from build123d import *

# Parameters (mm, degrees)
SKETCH2_W           = 50
SKETCH2_H           = 50
BOSS_EXTRUDE1_DEPTH = 3.175
SKETCH3_R           = 1.375
CUT_EXTRUDE1_DEPTH  = 36.497614356
SKETCH5_R           = 2.375
CUT_EXTRUDE3_DEPTH  = 1.9
CUT_EXTRUDE9_DEPTH  = 36.497614356
FILLET1_R           = 3
SKETCH11_W          = 15
SKETCH11_H          = 30
BOSS_EXTRUDE2_DEPTH = 3.175
CUT_EXTRUDE10_REACH = 62.499
CHAMFER1_SIZE       = 5


with BuildPart() as part:
    # Sketch2 → Boss-Extrude1 (new body)
    with BuildSketch(Plane(origin=(0, 0, 0), x_dir=(1, 0, 0), z_dir=(0, 1, 0))):
        Rectangle(SKETCH2_W, SKETCH2_H)
    extrude(amount=BOSS_EXTRUDE1_DEPTH)

    # Sketch3 → Cut-Extrude1 (cut, through all)
    with BuildSketch(Plane(origin=(0, 3.175, 0), x_dir=(1, 0, 0), z_dir=(0, 1, 0))):
        with Locations(Location((12.5, 12.5, 0), (0, 0, 270))):
            Circle(SKETCH3_R)
        with Locations(Location((-12.5, 12.5, 0), (0, 0, 270))):
            Circle(SKETCH3_R)
        with Locations(Location((-12.5, -12.5, 0), (0, 0, 270))):
            Circle(SKETCH3_R)
        with Locations(Location((12.5, -12.5, 0), (0, 0, 270))):
            Circle(SKETCH3_R)
    extrude(amount=-CUT_EXTRUDE1_DEPTH, mode=Mode.SUBTRACT)

    # Sketch5 → Cut-Extrude3 (cut)
    with BuildSketch(Plane.XZ):
        with Locations(Location((12.5, 12.5, 0), (0, 0, 270))):
            Circle(SKETCH5_R)
        with Locations(Location((-12.5, 12.5, 0), (0, 0, 270))):
            Circle(SKETCH5_R)
        with Locations(Location((12.5, -12.5, 0), (0, 0, 270))):
            Circle(SKETCH5_R)
        with Locations(Location((-12.5, -12.5, 0), (0, 0, 270))):
            Circle(SKETCH5_R)
    extrude(amount=-CUT_EXTRUDE3_DEPTH, mode=Mode.SUBTRACT)

    # Sketch10 → Cut-Extrude9 (cut, through all)
    with BuildSketch(Plane.XZ):
        Polygon((-9.25, -15.25), (9.25, -15.25), (9.25, -9.25), (15.25, -9.25), (15.25, 9.25), (9.25, 9.25), (9.25, 15.25), (-9.25, 15.25), (-9.25, 9.25), (-15.25, 9.25), (-15.25, -9.25), (-9.25, -9.25), align=None)
    extrude(amount=-CUT_EXTRUDE9_DEPTH, mode=Mode.SUBTRACT)

    # Fillet1
    fillet1_edges = [part.edges().sort_by_distance(p)[0] for p in [
        (15.25, 1.5875, -9.25),
        (15.25, 1.5875, 9.25),
        (-9.25, 1.5875, -15.25),
        (9.25, 1.5875, -15.25),
        (9.25, 1.5875, 15.25),
        (-9.25, 1.5875, 15.25),
        (-15.25, 1.5875, 9.25),
        (-15.25, 1.5875, -9.25),
        (9.25, 1.5875, 9.25),
        (-9.25, 1.5875, 9.25),
        (9.25, 1.5875, -9.25),
        (-9.25, 1.5875, -9.25),
    ]]
    fillet(fillet1_edges, radius=FILLET1_R - 0.0001)  # a hair under: the kernel refuses the full size

    # Sketch11 → Boss-Extrude2 (add)
    with BuildSketch(Plane(origin=(0, 3.175, 0), x_dir=(1, 0, 0), z_dir=(0, 1, 0))):
        with Locations((0, 40)):
            Rectangle(SKETCH11_W, SKETCH11_H)
    extrude(amount=-BOSS_EXTRUDE2_DEPTH)

    # Sketch13 → Cut-Extrude10 (cut, up to next)
    with BuildSketch(Plane(origin=(0, 3.175, 0), x_dir=(1, 0, 0), z_dir=(0, 1, 0)), mode=Mode.PRIVATE) as cut_extrude10_sk1:
        with BuildLine():
            Line((-3.05, 49.782863058), (-3.05, 21.813452658))
            ThreePointArc((-3.05, 21.813452658), (0, 18.763452658), (3.05, 21.813452658))
            Line((3.05, 21.813452658), (3.05, 49.782863058))
            ThreePointArc((3.05, 49.782863058), (0, 52.832863058), (-3.05, 49.782863058))
        make_face()
    cut_extrude10_tool1 = extrude(cut_extrude10_sk1.sketch, amount=-CUT_EXTRUDE10_REACH, mode=Mode.PRIVATE) & part.part
    add(cut_extrude10_tool1.solids().sort_by_distance((0, 3.175, -35.798158))[0], mode=Mode.SUBTRACT)

    # Chamfer1
    chamfer1_edges = [part.edges().sort_by_distance(p)[0] for p in [
        (7.5, 1.5875, -25),
        (7.5, 1.5875, -55),
        (-7.5, 1.5875, -55),
        (-7.5, 1.5875, -25),
        (25, 1.5875, 25),
        (-25, 1.5875, 25),
        (-25, 1.5875, -25),
        (25, 1.5875, -25),
    ]]
    chamfer(chamfer1_edges, length=CHAMFER1_SIZE)


solid = part.part
Build history of the part. All positions in model axes, mm. A direction names the side the tool comes from. Give positions to 0.01 mm unless a question says otherwise; leave off trailing zeros. Loops run counter-clockwise (first coordinate to the right, second up) from the corner with the lowest first, then second, coordinate; pieces in that order, holes last. Notation, with made-up numbers: (3, -26.75) - (56, -26.75) arc R24 cw to (56, -7.75) - close; hole circle Ø8 at (48.5, -35.75). An arc over 180 degrees is marked (long way). Write item = value, one per line. Start each with the question number.
1) Band-saw the part on C-C on y = 1.4. Count the separate pieces of the cut face and the enclosed holes in it, plus the area to 3 significant figures.
2) Pull direction X, two halves, no side cores. Call faces 4 (the flat face through (0, 2, 15.25)), 5 (the flat face through (7.5, 2, -40)), 6 (the flat face through (-22, 2, 23)): +X half, -X half, draft (parallel to the pull), parting line (faces both ways), or undercut.
3) Drop flat-ended pins along their axis: pin 1 Ø1 at (y, z) = (1.5, -35.5) entering from +X; pin 2 Ø2.5 at (x, z) = (-12, -12) entering from -Y; pin 3 Ø1.6 at (y, z) = (2, -42.5) entering from -X; pin 4 Ø1.4 at (x, z) = (-12, 12.5) entering from -Y. Give the stop position or say it passes through.
4) Probe probe 1 along X at (y, z) = (1.05, 12.5) (3 decimals); probe 2 along X at (y, z) = (2.6, 12.5) (3 decimals); probe 3 along X at (y, z) = (2.4, -30.5). List the from-to ranges inside material, lowest first. Write a range as from..to.
5) Tool access for faces 1 (the flat face through (-22, 2, -23)), 2 (the cylindrical face through (-8.39, 1.61, 14.35)), 3 (the cylindrical face through (14.5, 0.94, 11.22)): list every direction of +Z, -Z, +X, -X, +Y, -Y with a clear straight run to the whole face (end or side of a thin tool).
6) Band-saw the part on B-B on x = 4. Give the cut face in (y, z) (3 decimals).
7) Band-saw the part on A-A on z = -41. Give the cut face in (x, y) (3 decimals).
Final values:
q1.separate_pieces = 1
q1.enclosed_holes = 6
q1.area = 1,850 mm²
q2.face_4 = undercut
q2.face_5 = +X half
q2.face_6 = -X half
q3.pin_1 = 7.5
q3.pin_2 = 1.9
q3.pin_3 = -7.5
q3.pin_4 = through
q4.probe_1 = -25..-14.875, -10.125..-9.24, 9.24..10.125, 14.875..25
q4.probe_2 = -25..-13.875, -11.125..-9.24, 9.24..11.125, 13.875..25
q4.probe_3 = -7.5..-3.05, 3.05..7.5
q5.face_1 = -Z, -X, +Y, -Y
q5.face_2 = +Y, -Y
q5.face_3 = -Y
q6.outline = (0, -53.5) - (3.175, -53.5) - (3.175, -15.25) - (0, -15.25) - close; (0, 15.25) - (3.175, 15.25) - (3.175, 25) - (0, 25) - close
q7.outline = (-7.5, 0) - (-3.05, 0) - (-3.05, 3.175) - (-7.5, 3.175) - close; (3.05, 0) - (7.5, 0) - (7.5, 3.175) - (3.05, 3.175) - close
